For this review, take the finished solid that the model builds, in its own axes (mm). Coordinates: 2 decimals unless noted, no trailing zeros. Loops run counter-clockwise (first coordinate to the right, second up) from the corner with the lowest first, then second, coordinate; pieces in that order, holes last. Notation, with made-up numbers: (-3, 14) - (15, 14) arc R24 cw to (15, 48) - close; hole circle Ø10 at (75.5, -40). An arc over 180 degrees is marked (long way). Use one line per item in the form item = value. Start each with the question number.
1. To check wall thickness, follow probe 1 along X at (y, z) = (0, 2.7); probe 2 along Y at (x, z) = (-24.5, 4.3); probe 3 along Y at (x, z) = (-26, 3.75). State the ranges of each line that lie inside material, in increasing order.
2. Add section C-C on x = -24.5. Give the boundary of the cut face in (y, z).
3. Add section A-A on y = -10. Give the boundary of the cut face in (x, z).
4. For pin 1 Ø4.5 at (x, y) = (0, 22.225) entering from +Z; pin 2 Ø2 at (y, z) = (19, 5.5) entering from -X, all flat-tipped, find the tip position at first contact; note any pin that passes through.
5. Add section D-D on y = -16. Give the boundary of the cut face in (x, z), and give its area (3 significant figures).
6. Add section B-B on z = 5. Give the boundary of the cut face in (x, y) (3 decimals).
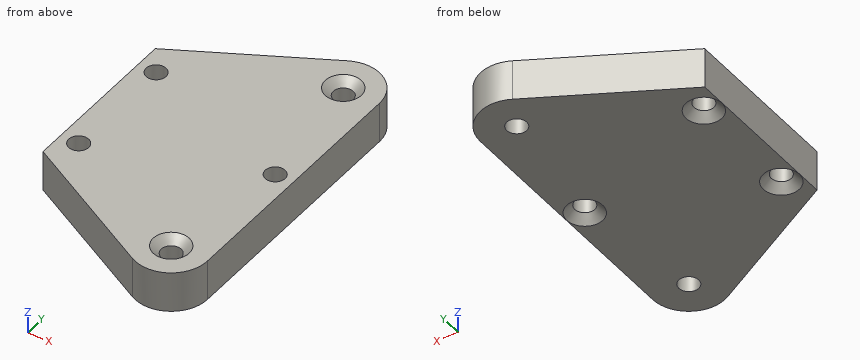
```python
from build123d import *

# Parameters (mm, degrees)
SKETCH1_R                                       = 1.75
BOSS_EXTRUDE1_DEPTH                             = 7.112
CSK_FOR_M3_FLAT_HEAD_MACHINE_SCREW1_D           = 3.2
CSK_FOR_M3_FLAT_HEAD_MACHINE_SCREW1_CSINK_D     = 6.3
CSK_FOR_M3_FLAT_HEAD_MACHINE_SCREW1_CSINK_ANGLE = 90
CSK_FOR_M3_FLAT_HEAD_MACHINE_SCREW2_D           = 3.2
CSK_FOR_M3_FLAT_HEAD_MACHINE_SCREW2_CSINK_D     = 6.3
CSK_FOR_M3_FLAT_HEAD_MACHINE_SCREW2_CSINK_ANGLE = 90
CSK_FOR_M3_FLAT_HEAD_MACHINE_SCREW3_D           = 3.2
CSK_FOR_M3_FLAT_HEAD_MACHINE_SCREW3_CSINK_D     = 6.3
CSK_FOR_M3_FLAT_HEAD_MACHINE_SCREW3_CSINK_ANGLE = 90


with BuildPart() as part:
    # Sketch1 → Boss-Extrude1 (new body)
    with BuildSketch(Plane.XY):
        with BuildLine():
            Line((-27.7, 14.5), (-27.7, -14.5))
            Line((-27.7, -14.5), (-3.014335177, -27.813942963))
            ThreePointArc((-3.014335177, -27.813942963), (3.254341072, -27.677684127), (6.35, -22.225))
            Line((6.35, -22.225), (6.35, 22.225))
            ThreePointArc((6.35, 22.225), (3.254341072, 27.677684127), (-3.014335177, 27.813942963))
            Line((-3.014335177, 27.813942963), (-27.7, 14.5))
        make_face()
        with Locations((0, 22.225)):
            Circle(SKETCH1_R, mode=Mode.SUBTRACT)
        with Locations((0, -22.225)):
            Circle(SKETCH1_R, mode=Mode.SUBTRACT)
        with Locations((-24.5, 10)):
            Circle(SKETCH1_R, mode=Mode.SUBTRACT)
        with Locations((-24.5, -10)):
            Circle(SKETCH1_R, mode=Mode.SUBTRACT)
        with Locations((3.15, 0)):
            Circle(SKETCH1_R, mode=Mode.SUBTRACT)
    extrude(amount=BOSS_EXTRUDE1_DEPTH)

    # CSK for M3 Flat Head Machine Screw1 (through all)
    with Locations(Plane(origin=(-24.5, 10, 0), x_dir=(-1, 0, 0), z_dir=(0, 0, -1))):
        with Locations((0, 0), (0, -20)):
            CounterSinkHole(CSK_FOR_M3_FLAT_HEAD_MACHINE_SCREW1_D / 2, CSK_FOR_M3_FLAT_HEAD_MACHINE_SCREW1_CSINK_D / 2, counter_sink_angle=CSK_FOR_M3_FLAT_HEAD_MACHINE_SCREW1_CSINK_ANGLE)

    # CSK for M3 Flat Head Machine Screw2 (through all)
    with Locations(Plane(origin=(0, 0, 0), x_dir=(-1, 0, 0), z_dir=(0, 0, -1))):
        with Locations((-3.15, 0)):
            CounterSinkHole(CSK_FOR_M3_FLAT_HEAD_MACHINE_SCREW2_D / 2, CSK_FOR_M3_FLAT_HEAD_MACHINE_SCREW2_CSINK_D / 2, counter_sink_angle=CSK_FOR_M3_FLAT_HEAD_MACHINE_SCREW2_CSINK_ANGLE)

    # CSK for M3 Flat Head Machine Screw3 (through all)
    with Locations(Plane.XY.offset(7.112)):
        with Locations((0, 22.225), (0, -22.225)):
            CounterSinkHole(CSK_FOR_M3_FLAT_HEAD_MACHINE_SCREW3_D / 2, CSK_FOR_M3_FLAT_HEAD_MACHINE_SCREW3_CSINK_D / 2, counter_sink_angle=CSK_FOR_M3_FLAT_HEAD_MACHINE_SCREW3_CSINK_ANGLE)


solid = part.part
```
Conclusion:
q1.probe_1 = -27.7 to 1.4, 4.9 to 6.35
q1.probe_2 = -16.23 to -11.75, -8.25 to 8.25, 11.75 to 16.23
q1.probe_3 = -15.42 to -10.9, -9.1 to 9.1, 10.9 to 15.42
q2.outline = (-16.23, 0) - (-13.15, 0) - (-11.75, 1.4) - (-11.75, 7.11) - (-16.23, 7.11) - close; (-8.25, 1.4) - (-6.85, 0) - (6.85, 0) - (8.25, 1.4) - (8.25, 7.11) - (-8.25, 7.11) - close; (11.75, 1.4) - (13.15, 0) - (16.23, 0) - (16.23, 7.11) - (11.75, 7.11) - close
q3.outline = (-27.7, 0) - (-27.65, 0) - (-26.25, 1.4) - (-26.25, 7.11) - (-27.7, 7.11) - close; (-22.75, 1.4) - (-21.35, 0) - (6.35, 0) - (6.35, 7.11) - (-22.75, 7.11) - close
q4.pin_1 = 6.21
q4.pin_2 = -21.21
q5.outline = (-24.92, 0) - (6.35, 0) - (6.35, 7.11) - (-24.92, 7.11) - close
q5.area = 222 mm^2
q6.outline = (-27.7, -14.5) - (-3.014, -27.814) arc R6.35 ccw to (6.35, -22.225) - (6.35, 22.225) arc R6.35 ccw to (-3.014, 27.814) - (-27.7, 14.5) - close; hole circle Ø3.5 at (-24.5, -10); hole circle Ø3.5 at (-24.5, 10); hole circle Ø3.5 at (0, -22.225); hole circle Ø3.5 at (0, 22.225); hole circle Ø3.5 at (3.15, 0)
